Autodesk Inventor part; units mm, degrees
sketch "Tampo_sketch" plane through (0, 0, 0) normal (0, 0, 1) x (1, 0, 0)
  line L0 (-800, 400) -> (800, 400)
  line L1 (800, 400) -> (800, -400)
  line L2 (800, -400) -> (-800, -400)
  line L3 (-800, -400) -> (-800, 400)
  line L4 (-800, 400) -> (800, -400) construction
  line L5 (800, 400) -> (-800, -400) construction
  point P0 (0, 0)
  point P1 (0, 0)
  dimension "d0" = 1600
  dimension "d1" = 800
extrude "Tampo_Extrusion" add sketch "Tampo_sketch" along normal mid plane 20
fillet "Fillet1" radius 3 12 edges at (800, 400, 0) (-800, 400, 0) (-800, -400, 0) (800, -400, 0) (0, -400, 10) (0, -400, -10) (800, 0, 10) (800, 0, -10) (-800, 0, 10) (-800, 0, -10) (0, 400, 10) (0, 400, -10)
sketch "perna_encaixe_Sketch2" plane through (0, 0, -10) normal (0, 0, -1) x (-1, 0, 0)
  line L0 (-674.8, 274.8) -> (-725.2, 274.8)
  line L1 (-725.2, 274.8) -> (-725.2, 325.2)
  line L2 (-725.2, 325.2) -> (-674.8, 325.2)
  line L3 (-674.8, 325.2) -> (-674.8, 274.8)
  line L4 (-674.8, 274.8) -> (-725.2, 325.2) construction
  line L5 (-725.2, 274.8) -> (-674.8, 325.2) construction
  point P0 (0, 0)
  point P1 (-700, 300)
  dimension "d5" = 300
  dimension "d6" = 700
  dimension "d7" = 50.4
extrude "perna_encaixe_rasgo" cut sketch "perna_encaixe_Sketch2" against normal blind 15
properties part number "Tampo" material "Wood (Oak)"
Input: part model. Units: mm. Frame: model coordinates. Round coordinates to 2 decimals unless told otherwise and drop trailing zeros. Loops run counter-clockwise (first coordinate to the right, second up) from the corner with the lowest first, then second, coordinate; pieces in that order, holes last. Notation, with made-up numbers: (37.5, -17.5) -> (52.5, -17.5) arc R12 ccw to (52.5, -10.5) -> close; hole circle Ø3 at (3, -30.75). An arc over 180 degrees is marked (long way). Use one line per item in the form item = value. Start each with the question number.
Item 1: Mould query, pull axis Z, two halves, no side actions, for faces 1 (the face through (-11, 6, 10)), 2 (the face through (-11, 6, -10)). Classes: pulls with the +Z half, pulls with the -Z half, needs draft (parallel to the pull), parting line crosses it, or undercut.
Item 2: Material intervals for L1, parallel to Y at x = 250, z = -8; L2, parallel to Y at x = -407.5, z = -8.25, sorted ascending. Write a range as from..to.
Item 3: Section query A-A on x = 703. Return the cut outline in (y, z).
Ans:
q1.face_1 = pulls with the +Z half
q1.face_2 = pulls with the -Z half
q2.L1 = -399.83..399.83
q2.L2 = -399.73..399.73
q3.outline = (-400, -7) arc R3 ccw to (-397, -10) -> (274.8, -10) -> (274.8, 5) -> (325.2, 5) -> (325.2, -10) -> (397, -10) arc R3 ccw to (400, -7) -> (400, 7) arc R3 ccw to (397, 10) -> (-397, 10) arc R3 ccw to (-400, 7) -> close
